The drawing under review shows one solid part. Ordinate dimensions are in mm from its lowest x, y, z. Round coordinates to 2 decimals unless told otherwise and drop trailing zeros. Order: outer loops, then holes, each group sorted by start corner. A loop starts at its lowest first (then second) coordinate and runs counter-clockwise, first axis right, second up. Notation, with made-up numbers: M 0,53 L 59,53 A25 cw 59,77 Z; hole C -38.5,-39.5 d10. An arc over 180 degrees is marked long. Answer as a JSON object with one key per item and string values. Group by question number.
1) To check wall thickness, follow line 1 (Y direction, x = 9, z = 2.3); line 2 (X direction, y = 5.5, z = 0.8); line 3 (X direction, y = 3.5, z = 1.9). State the ranges of each line that lie inside material, in increasing order.
2) Consider section A-A, the plane x = 9. Write out the cut boundary in (y, z).
3) Consider section C-C, the plane z = 0.6. Write out the cut boundary in (x, y).
4) Consider section D-D, the plane z = 2.1. Write out the cut boundary in (x, y), then the cut area to 3 significant figures.
5) The part is to be moulded in two halves that separate along Y. For the marked faces 1, 2 and 3, say which applies: +Y half, -Y half, draft (parallel to the pull), parting line (faces both ways), or undercut.
6) Consider section B-B, the plane y = 3.5. Write out the cut boundary in (x, z).
7) Insertion check: pin 1 Ø3 at (x, y) = (9, 3.5) entering from -Z. The pin has a flat end and moves straight along its axis. Give the tip position at first contact, or say it passes through.
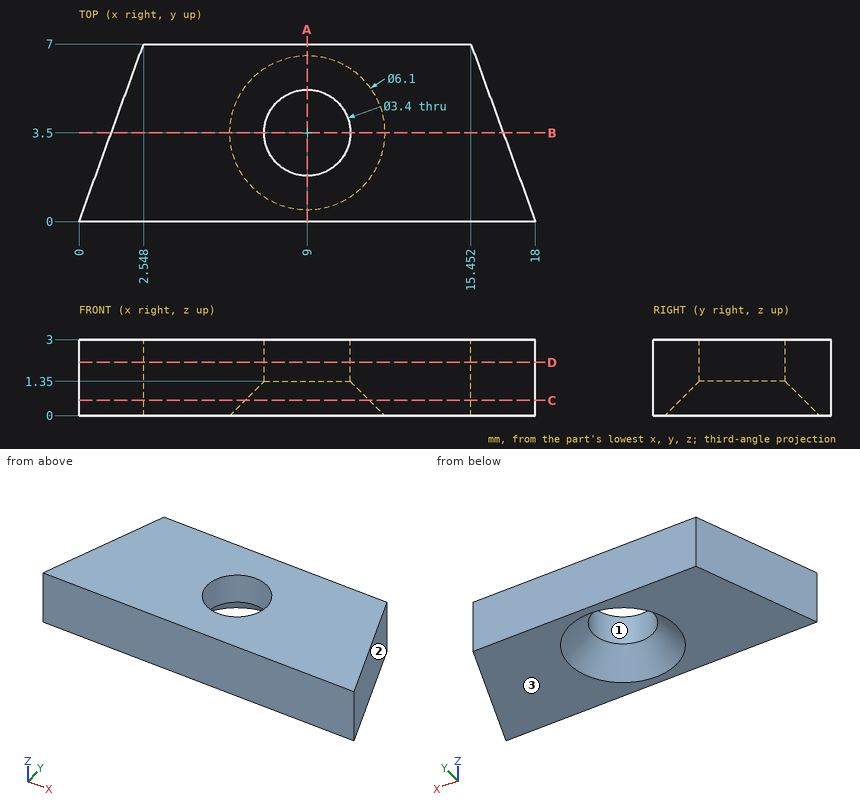
Results list:
{
 "1": {"line 1": "0 to 1.8, 5.2 to 7", "line 2": "2 to 7.97, 10.03 to 16", "line 3": "1.27 to 7.3, 10.7 to 16.73"},
 "2": {"outline": "M 0,0 L 0.45,0 L 1.8,1.35 L 1.8,3 L 0,3 Z; M 5.2,1.35 L 6.55,0 L 7,0 L 7,3 L 5.2,3 Z"},
 "3": {"outline": "M 0,0 L 18,0 L 15.45,7 L 2.55,7 Z; hole C 9,3.5 d4.9"},
 "4": {"outline": "M 0,0 L 18,0 L 15.45,7 L 2.55,7 Z; hole C 9,3.5 d3.4", "area": "99.1 mm^2"},
 "5": {"face 1": "undercut", "face 2": "+Y half", "face 3": "draft"},
 "6": {"outline": "M 1.27,0 L 5.95,0 L 7.3,1.35 L 7.3,3 L 1.27,3 Z; M 10.7,1.35 L 12.05,0 L 16.73,0 L 16.73,3 L 10.7,3 Z"},
 "7": {"pin 1": "through"}
}
